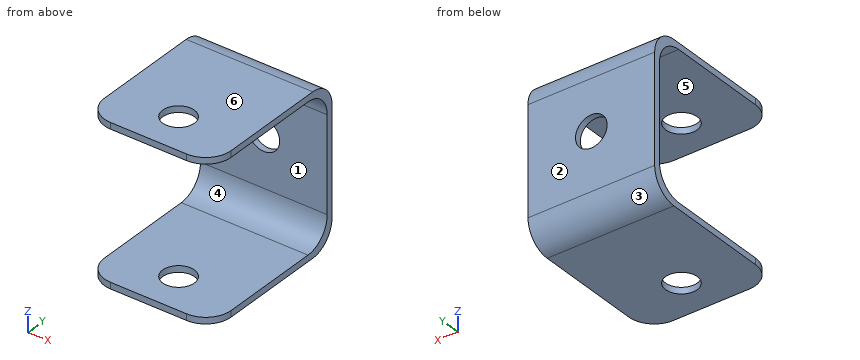
from build123d import *

# Parameters (mm, degrees)
F1_DEPTH      = 12.7
F1_DEPTH_BACK = 12.7
F2_R          = 3.175
F3_DEPTH      = 31.751
F4_R          = 5.08
F5_R          = 5.08
F6_R          = 3.175
F7_DEPTH      = 31.751


with BuildPart() as f1:
    # F0 (on Right) → F1 (new body, two sides)
    with BuildSketch(Plane.YZ) as f1_sk:
        Polygon((15.875, 15.875), (-15.875, 15.875), (-15.875, 14.605), (-14.605, 14.605), (14.605, 14.605), (14.605, -14.605), (-14.605, -14.605), (-15.875, -14.605), (-15.875, -15.875), (15.875, -15.875), align=None)
    extrude(amount=F1_DEPTH)
    extrude(f1_sk.sketch, amount=-F1_DEPTH_BACK)

    # F2 (on face) → F3 (cut, through all)
    with BuildSketch(Plane.XY.offset(15.875)):
        with Locations((0, -7.9502)):
            Circle(F2_R)
    extrude(amount=-F3_DEPTH, mode=Mode.SUBTRACT)

    # F4
    f4_edges = [f1.edges().sort_by_distance(p)[0] for p in [
        (0, 15.875, 15.875),
        (0, 15.875, -15.875),
        (0, 14.605, 14.605),
        (0, 14.605, -14.605),
    ]]
    fillet(f4_edges, radius=F4_R)

    # F5
    f5_edges = [f1.edges().sort_by_distance(p)[0] for p in [
        (12.7, -15.875, 15.24),
        (-12.7, -15.875, 15.24),
        (12.7, -15.875, -15.24),
        (-12.7, -15.875, -15.24),
    ]]
    fillet(f5_edges, radius=F5_R)

    # F6 (on face) → F7 (cut, through all)
    with BuildSketch(Plane(origin=(0, 15.875, 0), x_dir=(-1, 0, 0), z_dir=(0, 1, 0))):
        with Locations((0, 0.691243)):
            Circle(F6_R)
    extrude(amount=-F7_DEPTH, mode=Mode.SUBTRACT)


solid = f1.part
Verification items for the finished model (mm, model axes). Face numbers are marked on the shaded views. A direction names the side the tool comes from. Coordinates: 2 decimals unless noted, no trailing zeros. Order: outer loops, then holes, each group sorted by start corner. A loop starts at its lowest first (then second) coordinate and runs counter-clockwise, first axis right, second up.
Item 1: Access from +Z, -Z, +X, -X, +Y, -Y to the whole of each face (thin tool, end or side, straight path). Record for the marked faces 1 and 2.
Filled in:
face 1: +X, -X, -Y
face 2: +Z, -Z, +X, -X, +Y
Item 2: Section check D-D, the plane x = 2.75. Enter the section's corners in (y, z) (3 decimals).
Filled in:
outline: (-15.875, -15.875) - (-9.537, -15.875) - (-9.537, -14.605) - (-15.875, -14.605) - close; (-15.875, 14.605) - (-9.537, 14.605) - (-9.537, 15.875) - (-15.875, 15.875) - close; (-6.363, -15.875) - (10.795, -15.875) arc R5.08 ccw to (15.875, -10.795) - (15.875, -0.896) - (14.605, -0.896) - (14.605, -9.525) arc R5.08 cw to (9.525, -14.605) - (-6.363, -14.605) - close; (-6.363, 14.605) - (9.525, 14.605) arc R5.08 cw to (14.605, 9.525) - (14.605, 2.278) - (15.875, 2.278) - (15.875, 10.795) arc R5.08 ccw to (10.795, 15.875) - (-6.363, 15.875) - close
Item 3: Release check for a two-part mould opening along Z. For the marked faces 3, 4, 5 and 6 record: +Z half, -Z half, draft (parallel to the pull), parting line (faces both ways), or undercut.
Filled in:
face 3: -Z half
face 4: undercut
face 5: undercut
face 6: +Z half
Item 4: Material ranges on L1, parallel to Z at x = 11.5, y = -9.5 (3 decimals); L2, parallel to Y at x = 3.5, z = -1.5 (3 decimals); L3, parallel to Z at x = 0, y = 15.2, recorded low to high.
Filled in:
L1: z = -15.875 to -14.605, 14.605 to 15.875
L2: y = 14.605 to 15.875
L3: z = -13.33 to -2.48, 3.87 to 13.33
Item 5: Section check C-C, the plane z = -0.5. Enter the section's corners in (x, y) (3 decimals), then the cut area to 3 significant figures.
Filled in:
outline: (-12.7, 14.605) - (-2.943, 14.605) - (-2.943, 15.875) - (-12.7, 15.875) - close; (2.943, 14.605) - (12.7, 14.605) - (12.7, 15.875) - (2.943, 15.875) - close
area: 24.8 mm2
Item 6: Section check A-A, the plane y = -3.5. Enter the section's corners in (x, z) (3 decimals), then the cut area to 3 significant figures.
Filled in:
outline: (-12.7, -15.875) - (12.7, -15.875) - (12.7, -14.605) - (-12.7, -14.605) - close; (-12.7, 14.605) - (12.7, 14.605) - (12.7, 15.875) - (-12.7, 15.875) - close
area: 64.5 mm2
Item 7: Section check B-B, the plane x = 0. Enter the section's corners in (y, z) (3 decimals).
Filled in:
outline: (-15.875, -15.875) - (-11.125, -15.875) - (-11.125, -14.605) - (-15.875, -14.605) - close; (-15.875, 14.605) - (-11.125, 14.605) - (-11.125, 15.875) - (-15.875, 15.875) - close; (-4.775, -15.875) - (10.795, -15.875) arc R5.08 ccw to (15.875, -10.795) - (15.875, -2.484) - (14.605, -2.484) - (14.605, -9.525) arc R5.08 cw to (9.525, -14.605) - (-4.775, -14.605) - close; (-4.775, 14.605) - (9.525, 14.605) arc R5.08 cw to (14.605, 9.525) - (14.605, 3.866) - (15.875, 3.866) - (15.875, 10.795) arc R5.08 ccw to (10.795, 15.875) - (-4.775, 15.875) - close
Item 8: Depth check by flat-ended pin: pin 1 (4 mm diameter, centred on y = -5.5, z = 11.5, fed in from -X). Enter the tip coordinate at first touch or a pass-through.
Filled in:
pin 1: passes through
